from build123d import *

# Parameters (mm, degrees)
SKETCH1_W              = 30
SKETCH1_H              = 12.7
BOSS_EXTRUDE1_DEPTH    = 30
F_2_CLEARANCE_HOLE1_D  = 2.2606
SKETCH4_OUTSIDE_W      = 40.858
SKETCH4_OUTSIDE_H      = 40.858
SKETCH4_OUTSIDE_W_2    = 20
SKETCH4_OUTSIDE_H_2    = 30
CUT_EXTRUDE1_DEPTH     = 6.35
F_10_32_TAPPED_HOLE1_D = 4.0386


with BuildPart() as part:
    # Sketch1 → Boss-Extrude1 (new body)
    with BuildSketch(Plane.XY):
        with Locations((15, 6.35)):
            Rectangle(SKETCH1_W, SKETCH1_H)
    extrude(amount=BOSS_EXTRUDE1_DEPTH)

    # #2 Clearance Hole1 (through all)
    with Locations(Plane(origin=(0, 12.7, 0), x_dir=(1, 0, 0), z_dir=(0, 1, 0))):
        with Locations((2.5, -2.5), (27.5, -2.5), (27.5, -27.5), (2.5, -27.5)):
            Hole(F_2_CLEARANCE_HOLE1_D / 2)

    # Sketch4 outside → Cut-Extrude1 (cut)
    with BuildSketch(Plane(origin=(0, 12.7, 0), x_dir=(1, 0, 0), z_dir=(0, 1, 0))):
        with Locations((15, -15)):
            Rectangle(SKETCH4_OUTSIDE_W, SKETCH4_OUTSIDE_H)
        with Locations((15, -15)):
            Rectangle(SKETCH4_OUTSIDE_W_2, SKETCH4_OUTSIDE_H_2, mode=Mode.SUBTRACT)
    extrude(amount=-CUT_EXTRUDE1_DEPTH, mode=Mode.SUBTRACT)

    # #10-32 Tapped Hole1 (through all)
    with Locations(Plane(origin=(0, 12.7, 0), x_dir=(1, 0, 0), z_dir=(0, 1, 0))):
        with Locations((15, -3.8875), (15, -26.1125)):
            Hole(F_10_32_TAPPED_HOLE1_D / 2)


solid = part.part
Can you work these out from the model? Positions are in its coordinate system, mm. A direction names the side the tool comes from. Coordinates: 2 decimals unless noted, no trailing zeros. Write each loop counter-clockwise with the first axis right and the second up, starting at its lowest first coordinate (ties: lowest second). Pieces come first, ordered by that corner, then holes.
Q1. Imagine slicing it at B-B, the plane z = 18.75. List the corners of the cut face in (x, y) for me.
Results found:
outline: (0, 0) - (30, 0) - (30, 6.35) - (25, 6.35) - (25, 12.7) - (5, 12.7) - (5, 6.35) - (0, 6.35) - close
Q2. If we mould it in two halves opening along X, with no side actions, what happens to faces 3 (the face through (25, 10, 15)), 4 (the face through (28.63, 3.13, 27.45)), 5 (the face through (27, 6.35, 15))? For each: +X half, -X half, draft (parallel to the pull), parting line (faces both ways), or undercut.
Results found:
face 3: +X half
face 4: undercut
face 5: draft
Q3. Imagine slicing it at A-A, the plane x = 2.5. List the corners of the cut face in (y, z) for me.
Results found:
outline: (0, 0) - (6.35, 0) - (6.35, 1.37) - (0, 1.37) - close; (0, 3.63) - (6.35, 3.63) - (6.35, 26.37) - (0, 26.37) - close; (0, 28.63) - (6.35, 28.63) - (6.35, 30) - (0, 30) - close
Q4. For P1, Ø3, axis at y = 8.5, z = 3, coming from the -X side; P2, Ø1.5, axis at x = 28.5, z = 12, coming from the +Y side; P3, Ø5, axis at y = 9.5, z = 16.5, coming from the +X side, each with a flat end and sliding along its axis, tell me the tip position at first contact or that it passes through.
Results found:
P1: stops at x = 5
P2: stops at y = 6.35
P3: stops at x = 25
Q5. Imagine slicing it at C-C, the plane y = 9.5. List the corners of the cut face in (x, z) for me, plus the area to 3 significant figures.
Results found:
outline: (5, 0) - (25, 0) - (25, 30) - (5, 30) - close; hole circle Ø4.04 at (15, 3.89); hole circle Ø4.04 at (15, 26.11)
area: 574 mm2
Q6. Imagine slicing it at D-D, the plane x = 15. List the corners of the cut face in (y, z) for me.
Results found:
outline: (0, 0) - (12.7, 0) - (12.7, 1.87) - (0, 1.87) - close; (0, 5.91) - (12.7, 5.91) - (12.7, 24.09) - (0, 24.09) - close; (0, 28.13) - (12.7, 28.13) - (12.7, 30) - (0, 30) - close
Q7. Please list where these lines run through material, in increasing order: L1, parallel to Z at x = 15, y = 7.75; L2, parallel to Z at x = 2.5, y = 1.5; L3, parallel to X at y = 2, z = 27.5.
Results found:
L1: z = 0 to 1.87, 5.91 to 24.09, 28.13 to 30
L2: z = 0 to 1.37, 3.63 to 26.37, 28.63 to 30
L3: x = 0 to 1.37, 3.63 to 13.53, 16.47 to 26.37, 28.63 to 30
Q8. Which directions (+Z, -Z, +X, -X, +Y, -Y) give clear straight access to the entire face, cutting with the end or side of a thin tool? Please do faces 1 (the face through (2, 6.35, 15)), 2 (the face through (1.978, 3.131, 28.503)).
Results found:
face 1: +Z, -Z, -X, +Y
face 2: +Y, -Y
